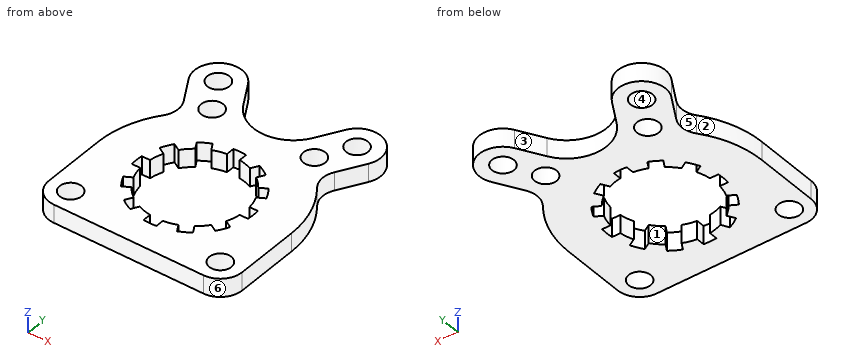
```python
from build123d import *

# Parameters (mm, degrees)
CROQUIS1_R              = 6
CROQUIS1_R_2            = 41
SALIENTE_EXTRUIR1_DEPTH = 10


with BuildPart() as part:
    # Croquis1 → Saliente-Extruir1 (new body)
    # profile 1 of 2: a face of its own
    with BuildSketch(Plane.XY):
        with BuildLine():
            ThreePointArc((49.258330249, 59.317930688), (44.5, 77.076260937), (26.741669751, 72.317930688))
            Line((26.741669751, 72.317930688), (19.052558883, 59))
            ThreePointArc((19.052558883, 59), (0, 48), (-19.052558883, 59))
            Line((-19.052558883, 59), (-26.741669751, 72.317930688))
            ThreePointArc((-26.741669751, 72.317930688), (-44.5, 77.076260937), (-49.258330249, 59.317930688))
            Line((-49.258330249, 59.317930688), (-41.258335188, 45.461532781))
            ThreePointArc((-41.258335188, 45.461532781), (-39.675518573, 38.68922066), (-42.115138595, 32.176327751))
            ThreePointArc((-42.115138595, 32.176327751), (-50.205097588, 16.983790583), (-53, 0))
            Line((-53, 0), (-53, -35))
            ThreePointArc((-53, -35), (-49.485281374, -43.485281374), (-41, -47))
            Line((-41, -47), (-9.521486782, -47))
            Line((-9.521486782, -47), (9.521486782, -47))
            Line((9.521486782, -47), (41, -47))
            ThreePointArc((41, -47), (49.485281374, -43.485281374), (53, -35))
            Line((53, -35), (53, 0))
            ThreePointArc((53, 0), (50.205097588, 16.983790583), (42.115138595, 32.176327751))
            ThreePointArc((42.115138595, 32.176327751), (39.675518573, 38.68922066), (41.258335188, 45.461532781))
            Line((41.258335188, 45.461532781), (49.258330249, 59.317930688))
        make_face()
        with Locations((-41, -35)):
            Circle(CROQUIS1_R, mode=Mode.SUBTRACT)
        with Locations((41, -35)):
            Circle(CROQUIS1_R, mode=Mode.SUBTRACT)
        Circle(CROQUIS1_R_2, mode=Mode.SUBTRACT)
        with Locations((-28, 48.497422612)):
            Circle(CROQUIS1_R, mode=Mode.SUBTRACT)
        with Locations((-38, 65.817930688)):
            Circle(CROQUIS1_R, mode=Mode.SUBTRACT)
        with Locations((28, 48.497422612)):
            Circle(CROQUIS1_R, mode=Mode.SUBTRACT)
        with Locations((38, 65.817930688)):
            Circle(CROQUIS1_R, mode=Mode.SUBTRACT)
    # profile 2 of 2: a face of its own
    with BuildSketch(Plane.XY):
        Circle(CROQUIS1_R_2)
        with BuildLine():
            ThreePointArc((10.607092784, 25.372023622), (7.11752374, 26.562960223), (3.5, 27.276363394))
            Line((3.5, 27.276363394), (3.5, 31.808017857))
            ThreePointArc((3.5, 31.808017857), (0, 32), (-3.5, 31.808017857))
            Line((-3.5, 31.808017857), (-3.5, 27.276363394))
            ThreePointArc((-3.5, 27.276363394), (-7.11752374, 26.562960223), (-10.607092784, 25.372023622))
            Line((-10.607092784, 25.372023622), (-12.872920015, 29.296551508))
            ThreePointArc((-12.872920015, 29.296551508), (-16, 27.712812921), (-18.935097842, 25.796551508))
            Line((-18.935097842, 25.796551508), (-16.66927061, 21.872023622))
            ThreePointArc((-16.66927061, 21.872023622), (-19.445436483, 19.445436483), (-21.872023622, 16.66927061))
            Line((-21.872023622, 16.66927061), (-25.796551508, 18.935097842))
            ThreePointArc((-25.796551508, 18.935097842), (-27.712812921, 16), (-29.296551508, 12.872920015))
            Line((-29.296551508, 12.872920015), (-25.372023622, 10.607092784))
            ThreePointArc((-25.372023622, 10.607092784), (-26.562960223, 7.11752374), (-27.276363394, 3.5))
            Line((-27.276363394, 3.5), (-31.808017857, 3.5))
            ThreePointArc((-31.808017857, 3.5), (-32, 0), (-31.808017857, -3.5))
            Line((-31.808017857, -3.5), (-27.276363394, -3.5))
            ThreePointArc((-27.276363394, -3.5), (-26.562960223, -7.11752374), (-25.372023622, -10.607092784))
            Line((-25.372023622, -10.607092784), (-29.296551508, -12.872920015))
            ThreePointArc((-29.296551508, -12.872920015), (-27.712812921, -16), (-25.796551508, -18.935097842))
            Line((-25.796551508, -18.935097842), (-21.872023622, -16.66927061))
            ThreePointArc((-21.872023622, -16.66927061), (-19.445436483, -19.445436483), (-16.66927061, -21.872023622))
            Line((-16.66927061, -21.872023622), (-18.935097842, -25.796551508))
            ThreePointArc((-18.935097842, -25.796551508), (-16, -27.712812921), (-12.872920015, -29.296551508))
            Line((-12.872920015, -29.296551508), (-10.607092784, -25.372023622))
            ThreePointArc((-10.607092784, -25.372023622), (-7.11752374, -26.562960223), (-3.5, -27.276363394))
            Line((-3.5, -27.276363394), (-3.5, -31.808017857))
            ThreePointArc((-3.5, -31.808017857), (0, -32), (3.5, -31.808017857))
            Line((3.5, -31.808017857), (3.5, -27.276363394))
            ThreePointArc((3.5, -27.276363394), (7.11752374, -26.562960223), (10.607092784, -25.372023622))
            Line((10.607092784, -25.372023622), (12.872920015, -29.296551508))
            ThreePointArc((12.872920015, -29.296551508), (16, -27.712812921), (18.935097842, -25.796551508))
            Line((18.935097842, -25.796551508), (16.66927061, -21.872023622))
            ThreePointArc((16.66927061, -21.872023622), (19.445436483, -19.445436483), (21.872023622, -16.66927061))
            Line((21.872023622, -16.66927061), (25.796551508, -18.935097842))
            ThreePointArc((25.796551508, -18.935097842), (27.712812921, -16), (29.296551508, -12.872920015))
            Line((29.296551508, -12.872920015), (25.372023622, -10.607092784))
            ThreePointArc((25.372023622, -10.607092784), (26.562960223, -7.11752374), (27.276363394, -3.5))
            Line((27.276363394, -3.5), (31.808017857, -3.5))
            ThreePointArc((31.808017857, -3.5), (32, 0), (31.808017857, 3.5))
            Line((31.808017857, 3.5), (27.276363394, 3.5))
            ThreePointArc((27.276363394, 3.5), (26.562960223, 7.11752374), (25.372023622, 10.607092784))
            Line((25.372023622, 10.607092784), (29.296551508, 12.872920015))
            ThreePointArc((29.296551508, 12.872920015), (27.712812921, 16), (25.796551508, 18.935097842))
            Line((25.796551508, 18.935097842), (21.872023622, 16.66927061))
            ThreePointArc((21.872023622, 16.66927061), (19.445436483, 19.445436483), (16.66927061, 21.872023622))
            Line((16.66927061, 21.872023622), (18.935097842, 25.796551508))
            ThreePointArc((18.935097842, 25.796551508), (16, 27.712812921), (12.872920015, 29.296551508))
            Line((12.872920015, 29.296551508), (10.607092784, 25.372023622))
        make_face(mode=Mode.SUBTRACT)
    extrude(amount=SALIENTE_EXTRUIR1_DEPTH)


solid = part.part
```
Read the model definition and answer for the solid it produces. Units are mm, in the model's axes. Face numbers are marked on the shaded views. A direction names the side the tool comes from. Give positions to 0.01 mm unless a question says otherwise; leave off trailing zeros. Order: outer loops, then holes, each group sorted by start corner. A loop starts at its lowest first (then second) coordinate and runs counter-clockwise, first axis right, second up.
(1) For a pull along X with two mould halves and no side action, classify the marked faces 4, 5 and 6 as released by +X, released by -X, zero draft, split by the parting line, or undercut.
(2) Find section B-B (x = -1.5). Give the vertices of the cut face in (y, z).
(3) Given pin 1 (11 mm diameter, centred on x = -28, y = 48.5, fed in from -Z); pin 2 (1.4 mm diameter, centred on y = 30, z = 5.5, fed in from -X); pin 3 (2.5 mm diameter, centred on x = -30, z = 3, fed in from +Y); pin 4 (1 mm diameter, centred on y = 7.5, z = 4.5, fed in from -X), each flat-ended and moving along its own axis, determine where each tip first touches the part or whether it passes through.
(4) For the marked faces 1, 2 and 3, determine the directions among +Z, -Z, +X, -X, +Y, -Y from which every point of the face is accessible in a straight line to the end or side of a thin tool.
(5) Find section C-C (z = 2). Give the number of separate pieces and of enclosed holes in the cut face, plus the area to 3 significant figures.
(6) Straight lines are drawn through the part: L1, parallel to X at y = -17, z = 7.5; L2, parallel to Y at x = -18.5, z = 5; L3, parallel to Y at x = -41, z = 4.75. For each, find the intervals that lie inside material, in ascending order.
(7) Find section A-A (x = -38). Give the vertices of the cut face in (y, z), plus the area to 3 significant figures.
Result sheet:
1. face 4: undercut
1. face 5: released by -X
1. face 6: released by +X
2. outline: (-47, 0) - (-31.96, 0) - (-31.96, 10) - (-47, 10) - close; (31.96, 0) - (48.05, 0) - (48.05, 10) - (31.96, 10) - close
3. pin 1: passes through
3. pin 2: stops at x = -44.16
3. pin 3: stops at y = 76.93
3. pin 4: stops at x = -52.54
4. face 1: +Z, -Z
4. face 2: +Z, -Z, -X
4. face 3: +Z, -Z, +Y
5. separate pieces: 1
5. enclosed holes: 7
5. area: 7,610 mm2
6. L1: x = -53 to -27.11, -22.44 to -21.62, 21.62 to 22.44, 27.11 to 53
6. L2: y = -47 to -26.11, -25.04 to -20.35, 20.35 to 25.04, 26.11 to 58.09
6. L3: y = -47 to -41, -29 to 33.93, 44.99 to 60.62, 71.01 to 78.47
7. outline: (-47, 0) - (-40.2, 0) - (-40.2, 10) - (-47, 10) - close; (-29.8, 0) - (59.82, 0) - (59.82, 10) - (-29.8, 10) - close; (71.82, 0) - (78.82, 0) - (78.82, 10) - (71.82, 10) - close
7. area: 1,030 mm2
